The figure shows three views and two pictorial views of one solid part (mm, origin at its lowest corner). Answer the questions. A direction names the side the tool comes from. Coordinates: 2 decimals unless noted, no trailing zeros. Order: outer loops, then holes, each group sorted by start corner. A loop starts at its lowest first (then second) coordinate and runs counter-clockwise, first axis right, second up. Notation, with made-up numbers: (-37.5, 15.25) -> (-21.5, 15.25) arc R33 ccw to (-21.5, 48.25) -> close; hole circle Ø4 at (86, 46). An arc over 180 degrees is marked (long way). Return JSON: item names as keys, results as strings.
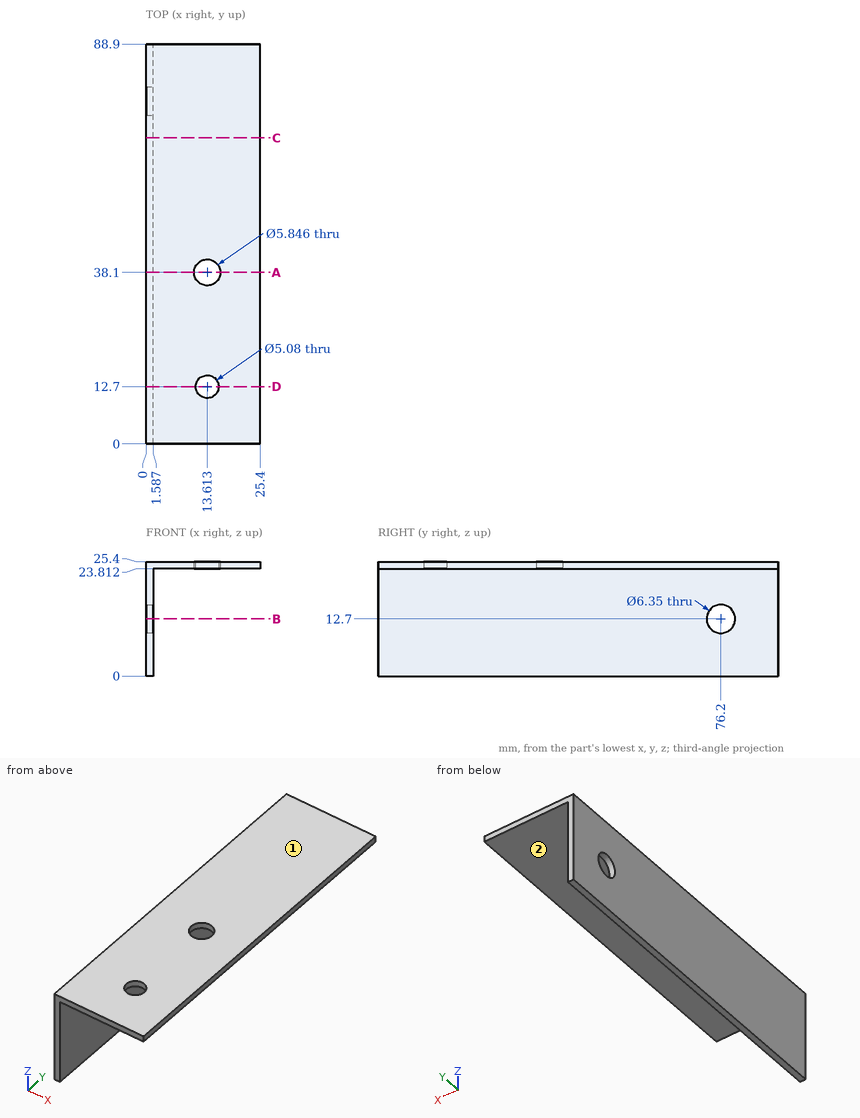
Item 1: The part is cut by section B-B on z = 12.7. Determine the outline of the cut face in (x, y) (1 decimal), plus the area to 3 significant figures.
Answer list:
{"outline": "(0, 0) -> (1.6, 0) -> (1.6, 73) -> (0, 73) -> close; (0, 79.4) -> (1.6, 79.4) -> (1.6, 88.9) -> (0, 88.9) -> close", "area": "131 mm2"}
Item 2: Which of the six approach directions +Z, -Z, +X, -X, +Y, -Y give full straight-line access (tool end or side, diameter ignored) to the marked faces 1 and 2?
Answer list:
{"face 1": "+Z, +X, -X, +Y, -Y", "face 2": "-Z, +X, +Y, -Y"}
Item 3: Flat-ended cylindrical pins translate along their axes: pin 1 (6 mm diameter, centred on y = 28, z = 19.5, fed in from +X); pin 2 (3 mm diameter, centred on x = 14, y = 53.5, fed in from -Z); pin 3 (10 mm diameter, centred on x = 7.5, z = 8, fed in from +Y); pin 4 (8.5 mm diameter, centred on y = 76.2, z = 12.7, fed in from -X). Find the tip coordinate at first contact, or state that the pin passes through.
Answer list:
{"pin 1": "x = 1.59", "pin 2": "z = 23.81", "pin 3": "through", "pin 4": "x = 0"}
Item 4: The part is cut by section D-D on y = 12.7. Determine the outline of the cut face in (x, z).
Answer list:
{"outline": "(0, 0) -> (1.59, 0) -> (1.59, 23.81) -> (11.07, 23.81) -> (11.07, 25.4) -> (0, 25.4) -> close; (16.15, 23.81) -> (25.4, 23.81) -> (25.4, 25.4) -> (16.15, 25.4) -> close"}
Item 5: The part is cut by section C-C on y = 68. Determine the outline of the cut face in (x, z).
Answer list:
{"outline": "(0, 0) -> (1.59, 0) -> (1.59, 23.81) -> (25.4, 23.81) -> (25.4, 25.4) -> (0, 25.4) -> close"}
Item 6: Find the intervals of material crossed by probe 1 along Y at (x, z) = (0.65, 12.7) (1 decimal); probe 2 along Z at (x, y) = (2.25, 57); probe 3 along X at (y, z) = (68, 10.25), in increasing order.
Answer list:
{"probe 1": "0 to 73, 79.4 to 88.9", "probe 2": "23.81 to 25.4", "probe 3": "0 to 1.59"}
Item 7: The part is cut by section A-A on y = 38.1. Determine the outline of the cut face in (x, z) (1 decimal).
Answer list:
{"outline": "(0, 0) -> (1.6, 0) -> (1.6, 23.8) -> (10.7, 23.8) -> (10.7, 25.4) -> (0, 25.4) -> close; (16.5, 23.8) -> (25.4, 23.8) -> (25.4, 25.4) -> (16.5, 25.4) -> close"}
